Build history of the part. All positions in model axes, mm. A direction names the side the tool comes from. Give positions to 0.01 mm unless a question says otherwise; leave off trailing zeros. Write each loop counter-clockwise with the first axis right and the second up, starting at its lowest first coordinate (ties: lowest second). Pieces come first, ordered by that corner, then holes. Notation, with made-up numbers: (53.5, 23) -> (74.5, 23) arc R27 cw to (74.5, 40) -> close; hole circle Ø1 at (-40, 89.25). An arc over 180 degrees is marked (long way). One line per question, with ' | ' between items. Start each with the question number.
(1) Pull direction Y, two halves, no side cores. Call faces 4 (the flat face through (-1, 30, 20)), 5 (the flat face through (10, -50, 38)), 6 (the flat face through (-10, 1, 60)), 7 (the flat face through (10, 50, 38)): released by +Y, released by -Y, zero draft, split by the parting line, or undercut.
(2) Band-saw the part on C-C, the plane y = 43. Give the cut face in (x, z), and give its area (3 significant figures).
(3) Tool access for faces 1 (the flat face through (30.876, -1, 80)), 2 (the flat face through (-1, -40, 0)), 3 (the flat face through (-1, -30, 20)): list every direction of +Z, -Z, +X, -X, +Y, -Y with a clear straight run to the whole face (end or side of a thin tool).
(4) Band-saw the part on B-B, the plane x = 33.5. Give the cut face in (y, z).
(5) Drill centre lines: probe 1 along Y at (x, z) = (24.5, 35); probe 2 along X at (y, z) = (39, 62); probe 3 along Z at (x, y) = (-26, -15). Where is each one in solid material? Low to high. Write a range as from..to.
(6) Band-saw the part on D-D, the plane z = 73. Give the cut face in (x, y), and give its area (3 significant figures).
(7) Pin check, flat tip, straight feed: P1, Ø1.5, axis at x = 25.5, y = -38, coming from the +Z side. Stop position of the tip, or through.
(8) Band-saw the part on A-A, the plane z = 23. Give the cut face in (x, y).
from build123d import *

# Parameters (mm, degrees)
F0_W     = 100
F0_H     = 100
F1_DEPTH = 100
F2_W     = 80.875554
F2_H     = 100
F3_DEPTH = 40
F4_W     = 60
F4_H     = 40
F5_DEPTH = 100.001


with BuildPart() as f1:
    # F0 (on Top) → F1 (new body)
    with BuildSketch(Plane.XY):
        Rectangle(F0_W, F0_H)
    extrude(amount=F1_DEPTH)

    # F2 (on face) → F3 (cut)
    with BuildSketch(Plane.XY.offset(100)):
        with Locations((-9.562223, 0)):
            Rectangle(F2_W, F2_H)
    extrude(amount=-F3_DEPTH, mode=Mode.SUBTRACT)

    # F4 (on face) → F5 (cut, through all)
    with BuildSketch(Plane(origin=(-50, 0, 0), x_dir=(0, -1, 0), z_dir=(-1, 0, 0))):
        with Locations((0, 20)):
            Rectangle(F4_W, F4_H)
    extrude(amount=-F5_DEPTH, mode=Mode.SUBTRACT)


solid = f1.part
Results:
1) face 4: undercut | face 5: released by -Y | face 6: zero draft | face 7: released by +Y
2) outline: (-50, 0) -> (50, 0) -> (50, 100) -> (30.88, 100) -> (30.88, 60) -> (-50, 60) -> close | area: 6,760 mm²
3) face 1: +Z, -X, +Y, -Y | face 2: -Z, +X, -X, +Y, -Y | face 3: -Z, +X, -X
4) outline: (-50, 0) -> (-30, 0) -> (-30, 40) -> (30, 40) -> (30, 0) -> (50, 0) -> (50, 100) -> (-50, 100) -> close
5) probe 1: y = -50..-30, 30..50 | probe 2: x = 30.88..50 | probe 3: z = 40..60
6) outline: (30.88, -50) -> (50, -50) -> (50, 50) -> (30.88, 50) -> close | area: 1,910 mm²
7) P1: stops at z = 60
8) outline: (-50, -50) -> (50, -50) -> (50, -30) -> (-50, -30) -> close; (-50, 30) -> (50, 30) -> (50, 50) -> (-50, 50) -> close
